For this review, use the dimensioned drawing (mm, ordinates from the lowest corner) and the shaded views. Round coordinates to 2 decimals unless told otherwise and drop trailing zeros. Loops run counter-clockwise (first coordinate to the right, second up) from the corner with the lowest first, then second, coordinate; pieces in that order, holes last. Notation, with made-up numbers: M 24,11.5 L 48,11.5 A26 ccw 48,42.5 Z; hole C 28.25,-1 d10. An arc over 180 degrees is marked long. Answer as a JSON object with one key per item and string values. Group by question number.
Item 1: Consider section B-B (y = 1). Give the boundary of the cut face in (x, z) (3 decimals).
Item 2: Consider section A-A (z = 3). Give the boundary of the cut face in (x, y) (3 decimals), and give its area (3 significant figures).
Item 3: To check wall thickness, follow line 1 (X direction, y = 2, z = 4.75). State the ranges of the line that lie inside material, in increasing order.
Item 4: Insertion check: P1, Ø1.2, axis at x = 53.625, z = 3, coming from the +Y side. The pin has a flat end and moves straight along its axis. Give the tip position at first contact, or say it passes through.
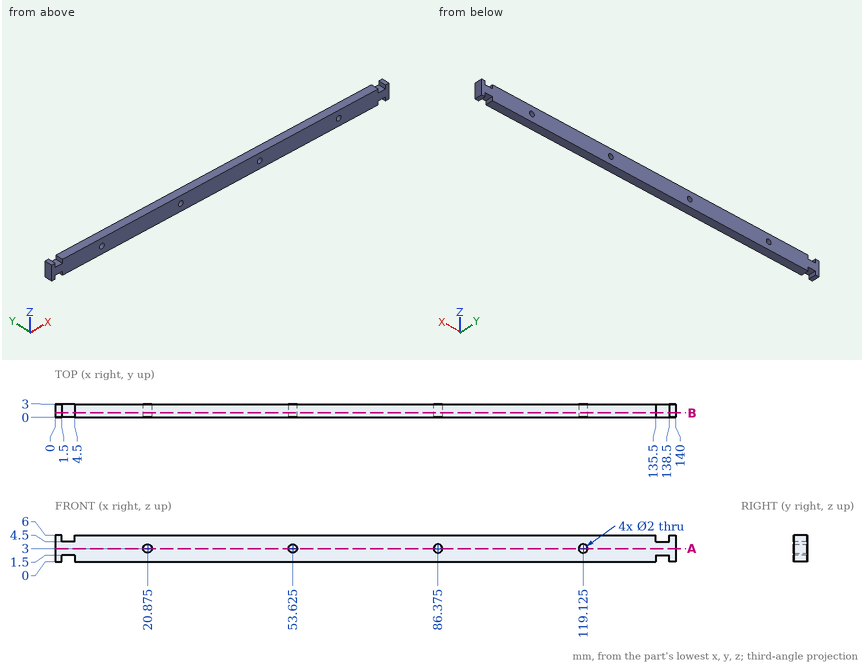
Geometry results:
{
 "1": {"outline": "M 0,0 L 1.5,0 L 1.5,1.5 L 4.5,1.5 L 4.5,0 L 135.5,0 L 135.5,1.5 L 138.5,1.5 L 138.5,0 L 140,0 L 140,6 L 138.5,6 L 138.5,4.5 L 135.5,4.5 L 135.5,6 L 4.5,6 L 4.5,4.5 L 1.5,4.5 L 1.5,6 L 0,6 Z; hole C 20.875,3 d2; hole C 53.625,3 d2; hole C 86.375,3 d2; hole C 119.125,3 d2"},
 "2": {"outline": "M 0,0 L 19.875,0 L 19.875,3 L 0,3 Z; M 21.875,0 L 52.625,0 L 52.625,3 L 21.875,3 Z; M 54.625,0 L 85.375,0 L 85.375,3 L 54.625,3 Z; M 87.375,0 L 118.125,0 L 118.125,3 L 87.375,3 Z; M 120.125,0 L 140,0 L 140,3 L 120.125,3 Z", "area": "396 mm^2"},
 "3": {"line 1": "x = 0 to 1.5, 4.5 to 135.5, 138.5 to 140"},
 "4": {"P1": "passes through"}
}
